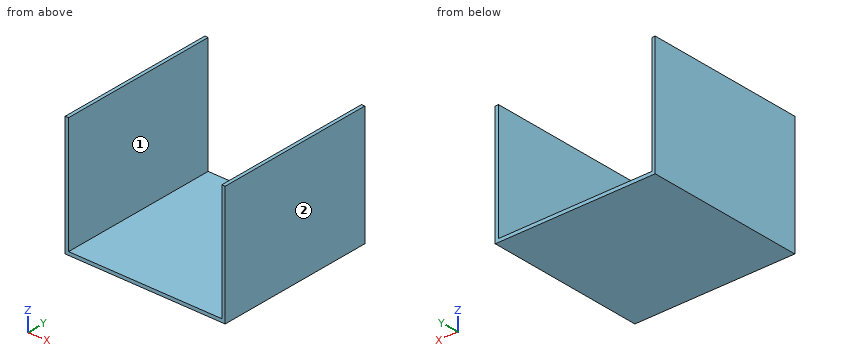
```python
from build123d import *

# Parameters (mm, degrees)
SKETCH1_W           = 609.6
SKETCH1_H           = 457.2
BOSS_EXTRUDE1_DEPTH = 609.6
SHELL1_T            = -12.7


with BuildPart() as part:
    # Sketch1 → Boss-Extrude1 (new body)
    with BuildSketch(Plane(origin=(0, 0, 0), x_dir=(1, 0, 0), z_dir=(0, 1, 0))):
        with Locations((304.8, 228.6)):
            Rectangle(SKETCH1_W, SKETCH1_H)
    extrude(amount=BOSS_EXTRUDE1_DEPTH)

    # Shell1
    shell1_openings = [part.faces().sort_by_distance(p)[0] for p in [
        (304.8, 609.6, -228.6),
        (304.8, 0, -228.6),
        (304.8, 304.8, 0),
    ]]
    offset(amount=SHELL1_T, openings=shell1_openings, kind=Kind.INTERSECTION)


solid = part.part
```
Design review of the part built by this model. Coordinates are the model's own, in mm. Face numbers are marked on the shaded views. A direction names the side the tool comes from. Give positions to 0.01 mm unless a question says otherwise; leave off trailing zeros. Order: outer loops, then holes, each group sorted by start corner. A loop starts at its lowest first (then second) coordinate and runs counter-clockwise, first axis right, second up. Notation, with made-up numbers: M 68.5,18.5 L 100.5,18.5 A6 cw 100.5,25.5 Z; hole C 70,-33 d10. An arc over 180 degrees is marked long. One line per question, with ' | ' between items. Start each with the question number.
Q1. Machinability: for the marked faces 1 and 2, which of the approach directions +Z, -Z, +X, -X, +Y, -Y give a long, thin tool a straight path to every point of the face, cutting with its end or side? Answer none if there is none.
Q2. We need section C-C (x = 285). Write out the cut boundary in (y, z), plus the area to 3 significant figures.
Q3. For L1, parallel to X at y = 555.5, z = -100; L2, parallel to Z at x = 112.5, y = 566, list the stretches that pass through material, from the lowest coordinate up. Write a range as [from, to].
Q4. We need section B-B (y = 377.5). Write out the cut boundary in (x, z).
Q5. We need section A-A (z = -403.5). Write out the cut boundary in (x, y), plus the area to 3 significant figures.
Q6. For pin 1 Ø1.5 at (y, z) = (508, -209) entering from -X, flat-tipped, find the tip position at first contact; note if it passes through.
Returned:
1) face 1: +Z, +Y, -Y | face 2: +Z, -Z, +X, +Y, -Y
2) outline: M 0,-457.2 L 609.6,-457.2 L 609.6,-444.5 L 0,-444.5 Z | area: 7,740 mm2
3) L1: [0, 12.7], [596.9, 609.6] | L2: [-457.2, -444.5]
4) outline: M 0,-457.2 L 609.6,-457.2 L 609.6,0 L 596.9,0 L 596.9,-444.5 L 12.7,-444.5 L 12.7,0 L 0,0 Z
5) outline: M 0,0 L 12.7,0 L 12.7,609.6 L 0,609.6 Z; M 596.9,0 L 609.6,0 L 609.6,609.6 L 596.9,609.6 Z | area: 15,500 mm2
6) pin 1: x = 0
